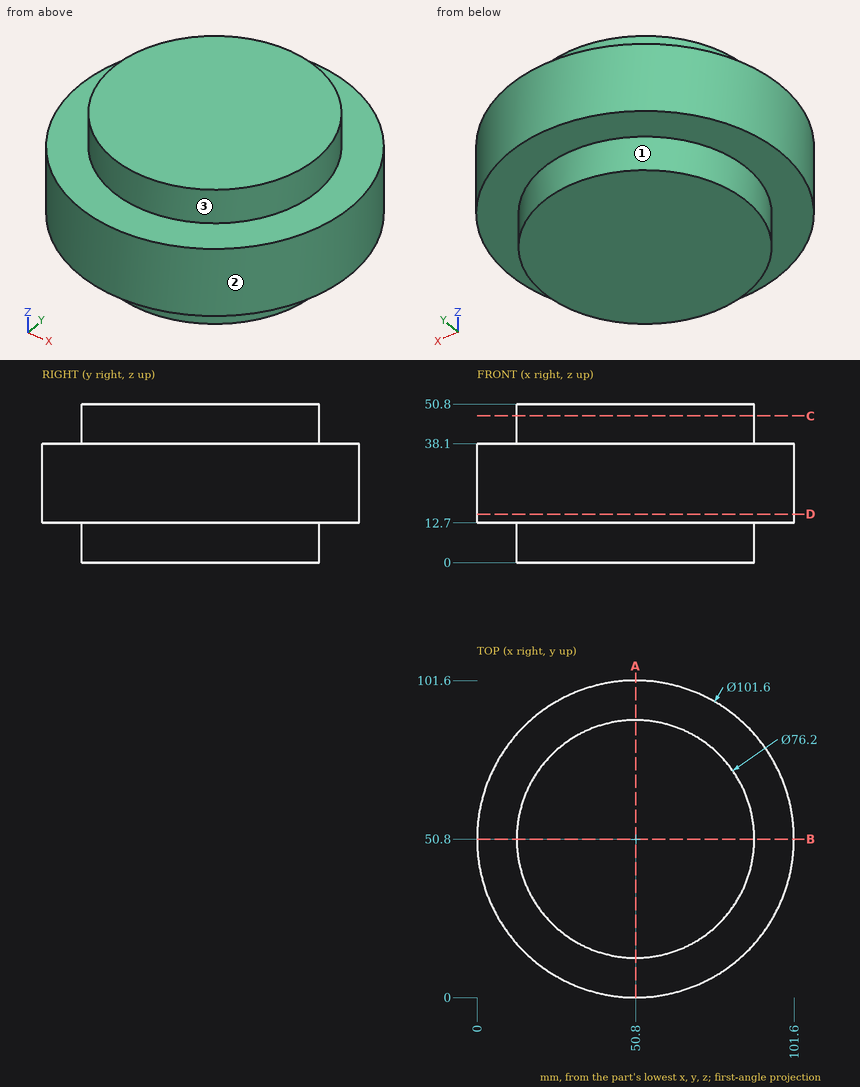
Geometry check sheet. Reference: drawing and pictorial views, mm from the part's lowest x, y, z. A direction names the side the tool comes from. Round coordinates to 2 decimals unless told otherwise and drop trailing zeros. Write each loop counter-clockwise with the first axis right and the second up, starting at its lowest first coordinate (ties: lowest second). Pieces come first, ordered by that corner, then holes.
Item 1: Section check C-C (z = 47). Record the boundary of the cut face in (x, y), plus the area to 3 significant figures.
Determined:
outline: circle Ø76.2 at (50.8, 50.8)
area: 4,560 mm2
Item 2: Section check A-A (x = 50.8). Record the boundary of the cut face in (y, z).
Determined:
outline: (0, 12.7) - (12.7, 12.7) - (12.7, 0) - (88.9, 0) - (88.9, 12.7) - (101.6, 12.7) - (101.6, 38.1) - (88.9, 38.1) - (88.9, 50.8) - (12.7, 50.8) - (12.7, 38.1) - (0, 38.1) - close
Item 3: Material ranges on line 1 along Z through (x, y) = (65, 9); line 2 along X through (y, z) = (8.5, 25.5); line 3 along Y through (x, z) = (47, 16), recorded low to high.
Determined:
line 1: z = 12.7 to 38.1
line 2: x = 22.67 to 78.93
line 3: y = 0.14 to 101.46
Item 4: Section check D-D (z = 15.5). Record the boundary of the cut face in (x, y).
Determined:
outline: circle Ø101.6 at (50.8, 50.8)
Item 5: Access from +Z, -Z, +X, -X, +Y, -Y to the whole of each face (thin tool, end or side, straight path). Record for the marked faces 1, 2 and 3.
Determined:
face 1: -Z
face 2: +Z, -Z
face 3: +Z
Item 6: Go/stop test with flat-tipped pins: pin 1 Ø3 at (x, z) = (90.5, 27) entering from -Y; pin 2 Ø3 at (y, z) = (37, 33.5) entering from +X; pin 3 Ø10 at (y, z) = (13, 7) entering from -X; pin 4 Ø6 at (x, y) = (70, 51.5) entering from -Z. Record where each tip stops, or that it passes through.
Determined:
pin 1: stops at y = 17.31
pin 2: stops at x = 100.09
pin 3: stops at x = 31.42
pin 4: stops at z = 0
